Can you work these out from the model? Positions are in its coordinate system, mm. A direction names the side the tool comes from. Round coordinates to 2 decimals unless told otherwise and drop trailing zeros. Write each loop counter-clockwise with the first axis right and the second up, starting at its lowest first coordinate (ties: lowest second). Pieces come first, ordered by that corner, then holes. Notation, with made-up numbers: (19, 80) -> (73, 80) arc R26 ccw to (73, 119) -> close; hole circle Ø4 at (-28.75, 47.25). An arc over 180 degrees is marked (long way). Write item = value, one per line. Start each with the question number.
1) Imagine slicing it at C-C, the plane x = -26.5. Please give me the cut outline in (y, z), then the cut area to 3 significant figures.
2) Imagine slicing it at B-B, the plane y = 3. State how many separate pieces and enclosed holes the cut face has, then the cut area to 3 significant figures.
3) I'm going to push flat-ended pins straight in: pin 1 (3 mm diameter, centred on x = -104, z = -7.5, fed in from +Y); pin 2 (4.5 mm diameter, centred on x = -26.5, z = -22.5, fed in from +Y). Where does each tip first touch, or does it pass through?
4) Imagine slicing it at A-A, the plane x = -60. Please give me the cut outline in (y, z).
5) Imagine slicing it at D-D, the plane z = -12.5. Please give me the cut outline in (x, y), then the cut area to 3 significant figures.
6) If I drill on line 1 (Z direction, x = -74.5, y = 3.85); line 2 (Z direction, x = -104, y = -1); line 3 (X direction, y = -5.75, z = -21), over which ranges is the centre line in solid material (lowest first)?
7) For faces 1 (the face through (-104, -12, -18)), 2 (the face through (-53, 0, -29)), 3 (the face through (-50, 3, -7)), which set-ups out of +Z, -Z, +X, -X, +Y, -Y let a thin tool reach every point of the face, with its end or its side?
Autodesk Inventor part; units mm, degrees
ref_plane "YZ Plane" through (0, 0, 0) normal (1, 0, 0) x (0, 1, 0)
ref_plane "XZ Plane" through (0, 0, 0) normal (0, 1, 0) x (-1, 0, 0)
ref_plane "XY Plane" through (0, 0, 0) normal (0, 0, 1) x (1, 0, 0)
sketch "Sketch1" plane through (0, 0, 0) normal (0, 1, 0) x (-1, 0, 0)
  line L0 (0, 0) -> (0, -35)
  line L1 (0, -35) -> (110, -35)
  line L2 (110, -35) -> (110, 0)
  line L3 (110, 0) -> (0, 0)
  line L4 (0, -35) -> (30, -35)
  line L5 (30, -17.5) -> (30, -28)
  line L6 (30, -28) -> (30, -7)
  line L7 (30, -7) -> (71, -7)
  line L8 (71, -7) -> (71, -28)
  line L9 (71, -28) -> (30, -28)
  circle A0 centre (74.5, -12.5) radius 2
  circle A1 centre (74.5, -22.5) radius 2
  circle A2 centre (26.5, -22.5) radius 2
  circle A3 centre (26.5, -12.5) radius 2
  dimension "d0" = 35
  dimension "d1" = 110
  dimension "d4" = 21
  dimension "d5" = 41
  dimension "d6" = 21
  dimension "d10" = 4
  dimension "d11" = 4
  dimension "d15" = 4
  dimension "d16" = 4
extrude "Extrusion1" add sketch "Sketch1" along normal blind 6
sketch "Sketch2" plane through (0, 0, -35) normal (0, 0, -1) x (-1, 0, 0)
  line L0 (0, 0) -> (0, 6)
  line L1 (0, 0) -> (0, -12)
  line L2 (22, -12) -> (22, 0)
  line L3 (0, 0) -> (110, 0)
  line L4 (22, -12) -> (18, -12)
  arc A0 (18, -12) -> (9.5, -12) centre (13.75, -12) ccw
  line L5 (9.5, -12) -> (0, -12)
  line L6 (110, 0) -> (110, -12)
  line L7 (85, -12) -> (85, 0)
  arc A1 (97.5, -12) -> (89, -12) centre (93.25, -12) ccw
  line L8 (89, -12) -> (85, -12)
  line L9 (110, -12) -> (97.5, -12)
  dimension "d19" = 12
  dimension "d20" = 22
  dimension "d21" = 4
  dimension "d23" = 8.5
  dimension "d24" = 12
  dimension "d25" = 25
  dimension "d26" = 8.5
  dimension "d27" = 8.25
extrude "Extrusion2" add sketch "Sketch2" against normal blind 35
sketch "Sketch3" plane through (-110, -12, -35) normal (0, -1, 0) x (1, 0, 0)
  line L0 (0, 0) -> (0, 35)
  circle A0 centre (6, 7.5) radius 2
  circle A1 centre (6, 27.5) radius 2
  line L1 (110, 35) -> (110, 0)
  circle A2 centre (105, 27.5) radius 2
  circle A3 centre (105, 7.5) radius 2
  dimension "d33" = 4
  dimension "d34" = 4
  dimension "d38" = 4
  dimension "d39" = 4
extrude "Extrusion3" cut sketch "Sketch3" against normal blind 18
properties part number "g_servo mount 1"
Reported:
q1.outline = (0, -35) -> (6, -35) -> (6, -24.5) -> (0, -24.5) -> close; (0, -20.5) -> (6, -20.5) -> (6, -14.5) -> (0, -14.5) -> close; (0, -10.5) -> (6, -10.5) -> (6, 0) -> (0, 0) -> close
q1.area = 162 mm²
q2.separate_pieces = 1
q2.enclosed_holes = 9
q2.area = 2,890 mm²
q3.pin_1 = through
q3.pin_2 = 6
q4.outline = (0, -35) -> (6, -35) -> (6, -28) -> (0, -28) -> close; (0, -7) -> (6, -7) -> (6, 0) -> (0, 0) -> close
q5.outline = (-110, -12) -> (-97.5, -12) arc R4.25 cw to (-89, -12) -> (-85, -12) -> (-85, 0) -> (-76.5, 0) -> (-76.5, 6) -> (-110, 6) -> close; (-72.5, 0) -> (-71, 0) -> (-71, 6) -> (-72.5, 6) -> close; (-30, 0) -> (-28.5, 0) -> (-28.5, 6) -> (-30, 6) -> close; (-24.5, 0) -> (-22, 0) -> (-22, -12) -> (-18, -12) arc R4.25 cw to (-9.5, -12) -> (0, -12) -> (0, 6) -> (-24.5, 6) -> close
q5.area = 873 mm²
q6.line_1 = -35 to -24.5, -20.5 to -14.5, -10.5 to 0
q6.line_2 = -35 to -29.5, -25.5 to -9.5, -5.5 to 0
q6.line_3 = -110 to -85, -22 to 0
q7.face_1 = +Z, -Z, +X, -X, -Y
q7.face_2 = +Z, -Z, -Y
q7.face_3 = +Y, -Y
